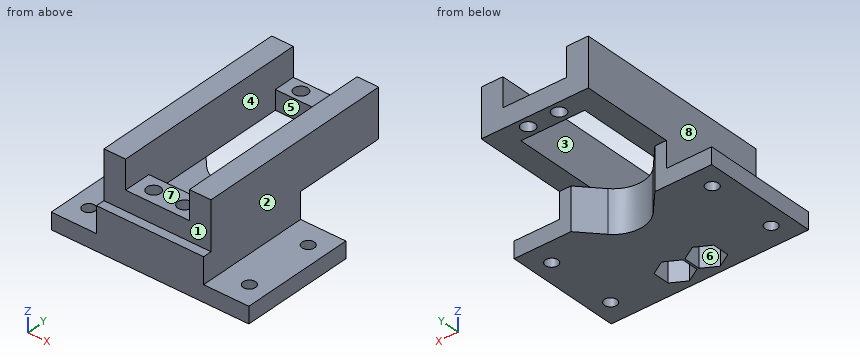
```python
from build123d import *

# Parameters (mm, degrees)
SZKIC1_W                    = 48
SZKIC1_H                    = 28
SZKIC1_R                    = 1.5
DODANIE_WYCI_GNI_CIE1_DEPTH = 4
WYTNIJ_WYCI_GNI_CIE1_DEPTH  = 4
SZKIC3_W                    = 26
SZKIC3_H                    = 6.7
DODANIE_WYCI_GNI_CIE2_DEPTH = 11
DODANIE_WYCI_GNI_CIE3_START = 6.3
DODANIE_WYCI_GNI_CIE3_DEPTH = 6.3
SZKIC5_W                    = 26
SZKIC5_H                    = 2.15
DODANIE_WYCI_GNI_CIE4_DEPTH = 6.3
DODANIE_WYCI_GNI_CIE7_DEPTH = 4.7
WYTNIJ_WYCI_GNI_CIE2_REACH  = 48.227
SZKIC10_R                   = 1.65
DODANIE_WYCI_GNI_CIE8_DEPTH = 7
WYTNIJ_WYCI_GNI_CIE3_DEPTH  = 7


with BuildPart() as part:
    # Szkic1 → Dodanie-wyciągnięcie1 (new body)
    with BuildSketch(Plane.XY):
        Rectangle(SZKIC1_W, SZKIC1_H)
        with Locations((-19.5, 8.5)):
            Circle(SZKIC1_R, mode=Mode.SUBTRACT)
        with Locations((-19.5, -8.5)):
            Circle(SZKIC1_R, mode=Mode.SUBTRACT)
        with Locations((19.5, -8.5)):
            Circle(SZKIC1_R, mode=Mode.SUBTRACT)
        with Locations((19.5, 8.5)):
            Circle(SZKIC1_R, mode=Mode.SUBTRACT)
    extrude(amount=DODANIE_WYCI_GNI_CIE1_DEPTH)

    # Szkic2 → Wytnij-wyciągnięcie1 (cut)
    with BuildSketch(Plane.XY.offset(4)):
        with BuildLine():
            Line((5.516782951, 8.919143195), (10.1961597, 14))
            Line((10.1961597, 14), (-10.1961597, 14))
            Line((-10.1961597, 14), (-5.516782951, 8.919143195))
            ThreePointArc((-5.516782951, 8.919143195), (0, 6.5), (5.516782951, 8.919143195))
        make_face()
    extrude(amount=-WYTNIJ_WYCI_GNI_CIE1_DEPTH, mode=Mode.SUBTRACT)

    # Szkic3 → Dodanie-wyciągnięcie2 (add)
    with BuildSketch(Plane.XY.offset(4)):
        with Locations((0, -8.5)):
            Rectangle(SZKIC3_W, SZKIC3_H)
    extrude(amount=DODANIE_WYCI_GNI_CIE2_DEPTH)

    # Szkic4 → Dodanie-wyciągnięcie3 (add)
    with BuildSketch(Plane.XY.offset(4).offset(DODANIE_WYCI_GNI_CIE3_START)):
        with BuildLine():
            Line((-13, -5.15), (13, -5.15))
            Line((13, -5.15), (13, 14))
            Line((13, 14), (10.1961597, 14))
            Line((10.1961597, 14), (5.516782951, 8.919143195))
            ThreePointArc((5.516782951, 8.919143195), (0, 6.5), (-5.516782951, 8.919143195))
            Line((-5.516782951, 8.919143195), (-10.1961597, 14))
            Line((-10.1961597, 14), (-13, 14))
            Line((-13, 14), (-13, -5.15))
        make_face()
    extrude(amount=-DODANIE_WYCI_GNI_CIE3_DEPTH)

    # Szkic5 → Dodanie-wyciągnięcie4 (add)
    with BuildSketch(Plane.XY.offset(4)):
        with Locations((0, -12.925)):
            Rectangle(SZKIC5_W, SZKIC5_H)
    extrude(amount=DODANIE_WYCI_GNI_CIE4_DEPTH)

    # Szkic9 → Dodanie-wyciągnięcie7 (add)
    with BuildSketch(Plane.XY.offset(10.3)):
        Polygon((-13, -5.15), (-13, 36.55), (13, 36.55), (13, -5.15), (7.75, -5.15), (7.75, 31.35), (-7.75, 31.35), (-7.75, -5.15), align=None)
    extrude(amount=DODANIE_WYCI_GNI_CIE7_DEPTH)

    # Wytnij-wyciągnięcie2: up to this face of the body (flat: up to its plane)
    wytnij_wyci_gni_cie2_end = Plane(part.part.faces().sort_by_distance((0, -0.888373191, 0))[0])
    # Szkic10 → Wytnij-wyciągnięcie2 (cut, up to the picked face)
    with BuildSketch(Plane.XY.offset(15), mode=Mode.PRIVATE) as wytnij_wyci_gni_cie2_sk1:
        with Locations((-3.75, -8.5)):
            Circle(SZKIC10_R)
    wytnij_wyci_gni_cie2_tool1 = split(extrude(wytnij_wyci_gni_cie2_sk1.sketch, amount=-WYTNIJ_WYCI_GNI_CIE2_REACH, mode=Mode.PRIVATE), bisect_by=wytnij_wyci_gni_cie2_end, keep=Keep.BOTH, mode=Mode.PRIVATE)
    # Szkic10 → Wytnij-wyciągnięcie2 (cut, up to the picked face)
    with BuildSketch(Plane.XY.offset(15), mode=Mode.PRIVATE) as wytnij_wyci_gni_cie2_sk2:
        with Locations((3.75, -8.5)):
            Circle(SZKIC10_R)
    wytnij_wyci_gni_cie2_tool2 = split(extrude(wytnij_wyci_gni_cie2_sk2.sketch, amount=-WYTNIJ_WYCI_GNI_CIE2_REACH, mode=Mode.PRIVATE), bisect_by=wytnij_wyci_gni_cie2_end, keep=Keep.BOTH, mode=Mode.PRIVATE)
    # Szkic10 → Wytnij-wyciągnięcie2 (cut, up to the picked face)
    with BuildSketch(Plane.XY.offset(15), mode=Mode.PRIVATE) as wytnij_wyci_gni_cie2_sk3:
        with Locations((-3.75, 34)):
            Circle(SZKIC10_R)
    wytnij_wyci_gni_cie2_tool3 = split(extrude(wytnij_wyci_gni_cie2_sk3.sketch, amount=-WYTNIJ_WYCI_GNI_CIE2_REACH, mode=Mode.PRIVATE), bisect_by=wytnij_wyci_gni_cie2_end, keep=Keep.BOTH, mode=Mode.PRIVATE)
    # Szkic10 → Wytnij-wyciągnięcie2 (cut, up to the picked face)
    with BuildSketch(Plane.XY.offset(15), mode=Mode.PRIVATE) as wytnij_wyci_gni_cie2_sk4:
        with Locations((3.75, 34)):
            Circle(SZKIC10_R)
    wytnij_wyci_gni_cie2_tool4 = split(extrude(wytnij_wyci_gni_cie2_sk4.sketch, amount=-WYTNIJ_WYCI_GNI_CIE2_REACH, mode=Mode.PRIVATE), bisect_by=wytnij_wyci_gni_cie2_end, keep=Keep.BOTH, mode=Mode.PRIVATE)
    add(wytnij_wyci_gni_cie2_tool1.solids().sort_by(Axis((-3.75, -8.5, 15), (0, 0, -1)))[0], mode=Mode.SUBTRACT)
    add(wytnij_wyci_gni_cie2_tool2.solids().sort_by(Axis((3.75, -8.5, 15), (0, 0, -1)))[0], mode=Mode.SUBTRACT)
    add(wytnij_wyci_gni_cie2_tool3.solids().sort_by(Axis((-3.75, 34, 15), (0, 0, -1)))[0], mode=Mode.SUBTRACT)
    add(wytnij_wyci_gni_cie2_tool4.solids().sort_by(Axis((3.75, 34, 15), (0, 0, -1)))[0], mode=Mode.SUBTRACT)

    # Szkic12 → Dodanie-wyciągnięcie8 (add)
    with BuildSketch(Plane.XY.offset(15)):
        Polygon((-7.75, 36.55), (-13, 36.55), (-13, -11.85), (-7.75, -11.85), (-7.75, -5.15), (-7.75, 31.35), align=None)
        Polygon((13, 36.55), (7.75, 36.55), (7.75, 31.35), (7.75, -5.15), (7.75, -11.85), (13, -11.85), align=None)
    extrude(amount=DODANIE_WYCI_GNI_CIE8_DEPTH)

    # Szkic14 → Wytnij-wyciągnięcie3 (cut)
    with BuildSketch(Plane(origin=(0, 0, 0), x_dir=(-1, 0, 0), z_dir=(0, 0, -1))):
        Polygon((-3.75, -4.458548116), (-7.25, -6.479274058), (-7.25, -10.520725942), (-3.75, -12.541451884), (-0.25, -10.520725942), (-0.25, -6.479274058), align=None)
        Polygon((3.75, -4.458548116), (0.25, -6.479274058), (0.25, -10.520725942), (3.75, -12.541451884), (7.25, -10.520725942), (7.25, -6.479274058), align=None)
    extrude(amount=-WYTNIJ_WYCI_GNI_CIE3_DEPTH, mode=Mode.SUBTRACT)


solid = part.part
```
Input: part model. Units: mm. Frame: model coordinates. Face numbers are marked on the shaded views. A direction names the side the tool comes from. Coordinates: 2 decimals unless noted, no trailing zeros. Order: outer loops, then holes, each group sorted by start corner. A loop starts at its lowest first (then second) coordinate and runs counter-clockwise, first axis right, second up. Notation, with made-up numbers: (34.25, 15) - (44.25, 15) arc R19 cw to (44.25, 22) - close; hole circle Ø11 at (-3.5, -21.75). An arc over 180 degrees is marked (long way). Put each result on its own line as item: value.
1. Cut plane A-A on x = 19.5. Return the cut outline in (y, z), then the cut area to 3 significant figures.
Report:
outline: (-14, 0) - (-10, 0) - (-10, 4) - (-14, 4) - close; (-7, 0) - (7, 0) - (7, 4) - (-7, 4) - close; (10, 0) - (14, 0) - (14, 4) - (10, 4) - close
area: 88.0 mm2
2. Cut plane C-C on z = 19. Return the cut outline in (x, y), then the cut area to 3 significant figures.
Report:
outline: (-13, -11.85) - (-7.75, -11.85) - (-7.75, 36.55) - (-13, 36.55) - close; (7.75, -11.85) - (13, -11.85) - (13, 36.55) - (7.75, 36.55) - close
area: 508 mm2
3. Reachability of the marked faces 4, 5, 6, 7 and 8 from +Z, -Z, +X, -X, +Y, -Y: full face, straight path, thin tool, end or side. Return the list, or none.
Report:
face 4: +Z
face 5: +Z, -Z
face 6: -Z
face 7: +Z, +Y, -Y
face 8: +Z, -X, +Y, -Y
4. Cut plane D-D on z = 5.25. Return the cut outline in (x, y).
Report:
outline: (-13, -14) - (13, -14) - (13, 14) - (10.2, 14) - (5.52, 8.92) arc R7.5 cw to (-5.52, 8.92) - (-10.2, 14) - (-13, 14) - close; hole (-7.25, -10.52) - (-3.75, -12.54) - (-0.25, -10.52) - (-0.25, -6.48) - (-3.75, -4.46) - (-7.25, -6.48) - close; hole (0.25, -10.52) - (3.75, -12.54) - (7.25, -10.52) - (7.25, -6.48) - (3.75, -4.46) - (0.25, -6.48) - close
5. Draft query along X for the marked faces 1, 2 and 3. Return one class per face: pulls with the +X half, pulls with the -X half, needs draft (parallel to the pull), parting line crosses it, or undercut.
Report:
face 1: needs draft
face 2: pulls with the +X half
face 3: undercut
6. Line query: line 1 along Y through (x, z) = (-3.75, 11.25); line 2 along Y through (x, z) = (-19.5, 1.7); line 3 along X through (y, z) = (-3.5, 13.75). Output: solid intervals per line, ascending.
Report:
line 1: y = -11.85 to -10.15, -6.85 to -5.15, 31.35 to 32.35, 35.65 to 36.55
line 2: y = -14 to -10, -7 to 7, 10 to 14
line 3: x = -13 to -7.75, 7.75 to 13
7. Cut plane B-B on y = 20. Return the cut outline in (x, z).
Report:
outline: (-13, 10.3) - (-7.75, 10.3) - (-7.75, 22) - (-13, 22) - close; (7.75, 10.3) - (13, 10.3) - (13, 22) - (7.75, 22) - close
8. Contact query for flat-ended pins moving along their axis: pin 1 Ø12 at (x, y) = (-4.5, 18.5) entering from -Z; pin 2 Ø11.5 at (x, z) = (-18.5, 6) entering from +Y; pin 3 Ø6 at (y, z) = (4, 18.5) entering from -X. Output: stop coordinate, or through.
Report:
pin 1: stops at z = 10.3
pin 2: stops at y = 14
pin 3: stops at x = -13
